Geometry: final body of the model. Coordinates: model frame, mm. A direction names the side the tool comes from. Give positions to 0.01 mm unless a question says otherwise; leave off trailing zeros. Write each loop counter-clockwise with the first axis right and the second up, starting at its lowest first coordinate (ties: lowest second). Pieces come first, ordered by that corner, then holes.
Q1. Mould query, pull axis Y, two halves, no side actions, for faces 3 (the flat face through (-31, -18, 15)), 4 (the cylindrical face through (40.49, -10.53, 91.48)), 5 (the cylindrical face through (41.504, -5.049, 91.479)). Classes: +Y half, -Y half, draft (parallel to the pull), parting line (faces both ways), or undercut.
Q2. Section D-D (x = 38.5). State how many separate pieces and enclosed holes the cut face has, plus the area to 3 significant figures.
Q3. Section A-A (z = 15.5). Return the cut outline in (x, y), plus the area to 3 significant figures.
Q4. Reachability of faces 1 (the flat face through (-33, -14, 105)), 2 (the cylindrical face through (-41.504, -5.049, 28.479)) from +Z, -Z, +X, -X, +Y, -Y: full face, straight path, thin tool, end or side. Return the list, or none.
Q5. Section B-B (y = -30). Return the cut outline in (x, z), plus the area to 3 significant figures.
Q6. Pin query (flat end, axial travel): pin 1 Ø5 at (y, z) = (-23, 86) entering from +X; pin 2 Ø10 at (y, z) = (-8.5, 101) entering from +X; pin 3 Ø6 at (y, z) = (-32, 99) entering from -X; pin 4 Ø6 at (x, z) = (-11.5, 44) entering from +Y. Return the tip coordinate at first contact, or that it passes through.
Q7. Section C-C (x = 21.5). Return the cut outline in (y, z).
Q8. Line query: line 1 (Y direction, x = -0.5, z = 30); line 2 (X direction, y = -32, z = 56.5); line 3 (X direction, y = -20, z = 101). Output: solid intervals per line, ascending.
from build123d import *

# Parameters (mm, degrees)
BOSS_EXTRUDE1_DEPTH = 120
SKETCH2_W           = 40.109469753
SKETCH2_H           = 60
SKETCH2_W_2         = 2
SKETCH2_H_2         = 20
CUT_EXTRUDE1_DEPTH  = 120
SKETCH3_R           = 5
SKETCH3_R_2         = 2
BOSS_EXTRUDE2_DEPTH = 3
BOSS_EXTRUDE3_START = -3
SKETCH4_R           = 5
SKETCH4_R_2         = 2
BOSS_EXTRUDE3_DEPTH = 3
LPATTERN1_COUNT     = 2
LPATTERN1_PITCH     = 90
FILLET1_R           = 60


with BuildPart() as part:
    # Sketch1 → Boss-Extrude1 (new body)
    with BuildSketch(Plane.XY):
        with BuildLine():
            ThreePointArc((33.80740392, -9.058666579), (0, -35), (-33.80740392, -9.058666579))
            ThreePointArc((-33.80740392, -9.058666579), (-35.032148792, -8.351559797), (-35.739255573, -9.576304669))
            ThreePointArc((-35.739255573, -9.576304669), (0, -37), (35.739255573, -9.576304669))
            ThreePointArc((35.739255573, -9.576304669), (35.032148792, -8.351559797), (33.80740392, -9.058666579))
        make_face()
    extrude(amount=BOSS_EXTRUDE1_DEPTH)

    # Sketch2 → Cut-Extrude1 (cut)
    with BuildSketch(Plane(origin=(0, 0, 0), x_dir=(1, 0, 0), z_dir=(0, 1, 0))):
        with Locations((-35.054734877, -60)):
            Rectangle(SKETCH2_W, SKETCH2_H)
        with Locations((35.054734877, -60)):
            Rectangle(SKETCH2_W, SKETCH2_H)
        with Locations((32, -15)):
            Rectangle(SKETCH2_W_2, SKETCH2_H_2)
        with Locations((-32, -15)):
            Rectangle(SKETCH2_W_2, SKETCH2_H_2)
        with Locations((-32, -105)):
            Rectangle(SKETCH2_W_2, SKETCH2_H_2)
        with Locations((32, -105)):
            Rectangle(SKETCH2_W_2, SKETCH2_H_2)
    extrude(amount=-CUT_EXTRUDE1_DEPTH, mode=Mode.SUBTRACT)

    # Sketch3 → Boss-Extrude2 (add)
    # profile 1 of 2: a face of its own
    with BuildSketch(Plane(origin=(0, 0, 0), x_dir=(-1, 0, 0), z_dir=(0, 0, -1))):
        with Locations((-38.899671742, -9.317485624)):
            Circle(SKETCH3_R)
        with Locations((-38.899671742, -9.317485624)):
            Circle(SKETCH3_R_2, mode=Mode.SUBTRACT)
    # profile 2 of 2: a face of its own
    with BuildSketch(Plane(origin=(0, 0, 0), x_dir=(-1, 0, 0), z_dir=(0, 0, -1))):
        with Locations((38.899671742, -9.317485624)):
            Circle(SKETCH3_R)
        with Locations(Location((38.899671742, -9.317485624, 0), (0, 0, 180))):
            Circle(SKETCH3_R_2, mode=Mode.SUBTRACT)
    boss_extrude2 = extrude(amount=-BOSS_EXTRUDE2_DEPTH)

    # Sketch4 → Boss-Extrude3 (add)
    # profile 1 of 2: a face of its own
    with BuildSketch(Plane.XY.offset(30).offset(BOSS_EXTRUDE3_START)):
        with Locations((-38.899671742, -9.317485624)):
            Circle(SKETCH4_R)
        with Locations((-38.899671742, -9.317485624)):
            Circle(SKETCH4_R_2, mode=Mode.SUBTRACT)
    # profile 2 of 2: a face of its own
    with BuildSketch(Plane.XY.offset(30).offset(BOSS_EXTRUDE3_START)):
        with Locations((38.899671742, -9.317485624)):
            Circle(SKETCH4_R)
        with Locations(Location((38.899671742, -9.317485624, 0), (0, 0, 180))):
            Circle(SKETCH4_R_2, mode=Mode.SUBTRACT)
    boss_extrude3 = extrude(amount=BOSS_EXTRUDE3_DEPTH)

    # LPattern1: Boss-Extrude2, Boss-Extrude3 ×2
    with Locations(*[(0, 0, i * LPATTERN1_PITCH) for i in range(1, LPATTERN1_COUNT)]):
        add(boss_extrude2)
        add(boss_extrude3)

    # Fillet1
    fillet1_edges = [part.edges().sort_by_distance(p)[0] for p in [
        (34.892782732, -12.308278238, 1.5),
        (-34.892782732, -12.308278238, 1.5),
        (-34.892782732, -12.308278238, 28.5),
        (34.892782732, -12.308278238, 28.5),
        (34.892782732, -12.308278238, 91.5),
        (-34.892782732, -12.308278238, 91.5),
        (-34.892782732, -12.308278238, 118.5),
        (34.892782732, -12.308278238, 118.5),
    ]]
    fillet(fillet1_edges, radius=FILLET1_R)


solid = part.part
Computed:
1. face 3: draft
1. face 4: undercut
1. face 5: parting line
2. separate pieces: 8
2. enclosed holes: 0
2. area: 86.3 mm2
3. outline: (-35.74, -9.58) arc R37 ccw to (-33, -16.73) - (-33, -11.66) arc R35 cw to (-33.81, -9.06) arc R1 ccw to start; (-31, -20.2) arc R37 ccw to (31, -20.2) - (31, -16.25) arc R35 cw to (-31, -16.25) - close; (33, -16.73) arc R37 ccw to (35.74, -9.58) arc R1 ccw to (33.81, -9.06) arc R35 cw to (33, -11.66) - close
3. area: 174 mm2
4. face 1: +Y, -Y
4. face 2: +Z, -Z
5. outline: (-21.66, 0) - (-18.03, 0) - (-18.03, 30) - (-21.66, 30) - close; (-21.66, 90) - (-18.03, 90) - (-18.03, 120) - (-21.66, 120) - close; (18.03, 0) - (21.66, 0) - (21.66, 30) - (18.03, 30) - close; (18.03, 90) - (21.66, 90) - (21.66, 120) - (18.03, 120) - close
5. area: 435 mm2
6. pin 1: passes through
6. pin 2: stops at x = 35.77
6. pin 3: stops at x = -22.98
6. pin 4: stops at y = -31.86
7. outline: (-30.11, 0) - (-27.62, 0) - (-27.62, 30) - (-30.11, 30) - close; (-30.11, 90) - (-27.62, 90) - (-27.62, 120) - (-30.11, 120) - close
8. line 1: y = -37 to -35
8. line 2: x = -15 to -14.18, 14.18 to 15
8. line 3: x = -31 to -28.72, 28.72 to 31
